Work out the finished part from the listing and answer in its coordinate system (mm). Give positions to 0.01 mm unless a question says otherwise; leave off trailing zeros. Loops run counter-clockwise (first coordinate to the right, second up) from the corner with the lowest first, then second, coordinate; pieces in that order, holes last.
from build123d import *

# Parameters (mm, degrees)
SPLIT_START       = 45
SPLIT_1_OUTLINE_W = 90
SPLIT_1_OUTLINE_H = 100
SPLIT_1_DEPTH     = 10
SKETCH_1_W        = 90
SKETCH_1_H        = 50
EXTRUDE_1_DEPTH   = 10


# Read off the part's stored shape, not the designer's step: 基材零件-專題-1
with BuildPart() as part:
    # Split 1 outline → Split 1 (new body)
    with BuildSketch(Plane.XY.offset(SPLIT_START)):
        with Locations((0, -42)):
            Rectangle(SPLIT_1_OUTLINE_W, SPLIT_1_OUTLINE_H)
        with BuildLine():
            Line((-40, -84), (-40, -54))
            ThreePointArc((-40, -54), (-35, -49), (-30, -54))
            Line((-30, -54), (-30, -84))
            ThreePointArc((-30, -84), (-35, -89), (-40, -84))
        make_face(mode=Mode.SUBTRACT)
        with BuildLine():
            Line((-25, -73), (-25, -48))
            ThreePointArc((-25, -48), (-21.75, -44.75), (-18.5, -48))
            Line((-18.5, -48), (-18.5, -73))
            ThreePointArc((-18.5, -73), (-21.75, -76.25), (-25, -73))
        make_face(mode=Mode.SUBTRACT)
        with BuildLine():
            Line((30, -84), (30, -54))
            ThreePointArc((30, -54), (35, -49), (40, -54))
            Line((40, -54), (40, -84))
            ThreePointArc((40, -84), (35, -89), (30, -84))
        make_face(mode=Mode.SUBTRACT)
        with BuildLine():
            Line((18.5, -73), (18.5, -48))
            ThreePointArc((18.5, -48), (21.75, -44.75), (25, -48))
            Line((25, -48), (25, -73))
            ThreePointArc((25, -73), (21.75, -76.25), (18.5, -73))
        make_face(mode=Mode.SUBTRACT)
        with BuildLine():
            Line((-18.5, -11), (-18.5, -36))
            ThreePointArc((-18.5, -36), (-21.75, -39.25), (-25, -36))
            Line((-25, -36), (-25, -11))
            ThreePointArc((-25, -11), (-21.75, -7.75), (-18.5, -11))
        make_face(mode=Mode.SUBTRACT)
        with BuildLine():
            ThreePointArc((-30, -30), (-35, -35), (-40, -30))
            Line((-40, -30), (-40, 0))
            ThreePointArc((-40, 0), (-35, 5), (-30, 0))
            Line((-30, 0), (-30, -30))
        make_face(mode=Mode.SUBTRACT)
        with BuildLine():
            Line((25, -11), (25, -36))
            ThreePointArc((25, -36), (21.75, -39.25), (18.5, -36))
            Line((18.5, -36), (18.5, -11))
            ThreePointArc((18.5, -11), (21.75, -7.75), (25, -11))
        make_face(mode=Mode.SUBTRACT)
        with BuildLine():
            ThreePointArc((40, -30), (35, -35), (30, -30))
            Line((30, -30), (30, 0))
            ThreePointArc((30, 0), (35, 5), (40, 0))
            Line((40, 0), (40, -30))
        make_face(mode=Mode.SUBTRACT)
    extrude(amount=SPLIT_1_DEPTH)

    # 草圖1 → 填料-伸長1 (add)
    with BuildSketch(Plane.XY.offset(55)):
        with Locations((0, -117)):
            Rectangle(SKETCH_1_W, SKETCH_1_H)
        with BuildLine():
            Line((40, -134), (40, -104))
            ThreePointArc((40, -104), (35, -99), (30, -104))
            Line((30, -104), (30, -134))
            ThreePointArc((30, -134), (35, -139), (40, -134))
        make_face(mode=Mode.SUBTRACT)
        with BuildLine():
            Line((25, -123), (25, -98))
            ThreePointArc((25, -98), (21.75, -94.75), (18.5, -98))
            Line((18.5, -98), (18.5, -123))
            ThreePointArc((18.5, -123), (21.75, -126.25), (25, -123))
        make_face(mode=Mode.SUBTRACT)
        with BuildLine():
            Line((-18.5, -123), (-18.5, -98))
            ThreePointArc((-18.5, -98), (-21.75, -94.75), (-25, -98))
            Line((-25, -98), (-25, -123))
            ThreePointArc((-25, -123), (-21.75, -126.25), (-18.5, -123))
        make_face(mode=Mode.SUBTRACT)
        with BuildLine():
            Line((-40, -134), (-40, -104))
            ThreePointArc((-40, -104), (-35, -99), (-30, -104))
            Line((-30, -104), (-30, -134))
            ThreePointArc((-30, -134), (-35, -139), (-40, -134))
        make_face(mode=Mode.SUBTRACT)
    extrude(amount=-EXTRUDE_1_DEPTH)


solid = part.part
Item 1: Find section D-D, the plane z = 52.5. Give the number of separate pieces and of enclosed holes in the cut face, plus the area to 3 significant figures.
Item 2: Find section A-A, the plane y = -79.5. Write down the section's boundary in (x, z).
Item 3: Determine the mould class of faces 1 (the face through (45, -68, 50)), 2 (the face through (21.82, -39.25, 49.93)), 3 (the face through (-1, 8, 50)), 4 (the face through (-25, -110, 50)) for opening direction X: released by +X, released by -X, zero draft, split by the parting line, or undercut.
Item 4: Find section C-C, the plane y = -120. Write down the section's boundary in (x, z).
Item 5: Consider line 1 (X direction, y = -103.5, z = 52.5); line 2 (X direction, y = -6.5, z = 53.5); line 3 (X direction, y = -45.5, z = 50.25). Determine where each line is inside the solid, lowest interval first.
Item 6: Find section B-B, the plane x = 35. Write down the section's boundary in (y, z), plus the area to 3 significant figures.
Ans:
1. separate pieces: 1
1. enclosed holes: 12
1. area: 10,100 mm2
2. outline: (-45, 45) - (-40, 45) - (-40, 55) - (-45, 55) - close; (-30, 45) - (30, 45) - (30, 55) - (-30, 55) - close; (40, 45) - (45, 45) - (45, 55) - (40, 55) - close
3. face 1: released by +X
3. face 2: undercut
3. face 3: zero draft
3. face 4: undercut
4. outline: (-45, 45) - (-40, 45) - (-40, 55) - (-45, 55) - close; (-30, 45) - (-25, 45) - (-25, 55) - (-30, 55) - close; (-18.5, 45) - (18.5, 45) - (18.5, 55) - (-18.5, 55) - close; (25, 45) - (30, 45) - (30, 55) - (25, 55) - close; (40, 45) - (45, 45) - (45, 55) - (40, 55) - close
5. line 1: x = -45 to -39.97, -30.03 to -25, -18.5 to 18.5, 25 to 30.03, 39.97 to 45
5. line 2: x = -45 to -40, -30 to 30, 40 to 45
5. line 3: x = -45 to -23.83, -19.67 to 19.67, 23.83 to 45
6. outline: (-142, 45) - (-139, 45) - (-139, 55) - (-142, 55) - close; (-99, 45) - (-89, 45) - (-89, 55) - (-99, 55) - close; (-49, 45) - (-35, 45) - (-35, 55) - (-49, 55) - close; (5, 45) - (8, 45) - (8, 55) - (5, 55) - close
6. area: 300 mm2
